Print and shaded views of the part. All mm, measured from the part's lowest x, y and z. A direction names the side the tool comes from. Round coordinates to 2 decimals unless told otherwise and drop trailing zeros. Order: outer loops, then holes, each group sorted by start corner. A loop starts at its lowest first (then second) coordinate and runs counter-clockwise, first axis right, second up. Notation, with made-up numbers: M 61.25,14 L 101.25,14 A12 cw 101.25,34 Z; hole C -38,32 d6. An arc over 180 degrees is marked long. Write each question's results on one line, items separated by ' | '. Start each with the question number.
1. Probe L1, parallel to X at y = 9.5, z = 2.5; L2, parallel to Y at x = 3.75, z = 1.25; L3, parallel to X at y = 0.2, z = 3.5 (1 decimal). List the from-to ranges inside material, lowest first. Write a range as [from, to].
2. Band-saw the part on B-B, the plane x = 5.75. List the corners of the cut face in (y, z).
3. Which spindle directions (+Z, -Z, +X, -X, +Y, -Y) get a long thin tool onto all of the face, cutting with end or side? Do the marked faces 5 and 6. Say none if no direction does.
4. Band-saw the part on D-D, the plane z = 0.5. List the corners of the cut face in (x, y).
5. Drop flat-ended pins along their axis: pin 1 Ø3.5 at (y, z) = (7, 2.5) entering from -X; pin 2 Ø3 at (x, z) = (3, 5) entering from +Y; pin 3 Ø1 at (x, y) = (6.5, 3.5) entering from +Z. Give the stop position or say it passes through.
6. Band-saw the part on C-C, the plane y = 12.25. List the corners of the cut face in (x, z).
7. Band-saw the part on A-A, the plane y = 8. List the corners of the cut face in (x, z).
8. Two-plate mould, pull along X, no slides. Class the marked faces 1, 2, 3 and 4: +X half, -X half, draft (parallel to the pull), parting line (faces both ways), or undercut.
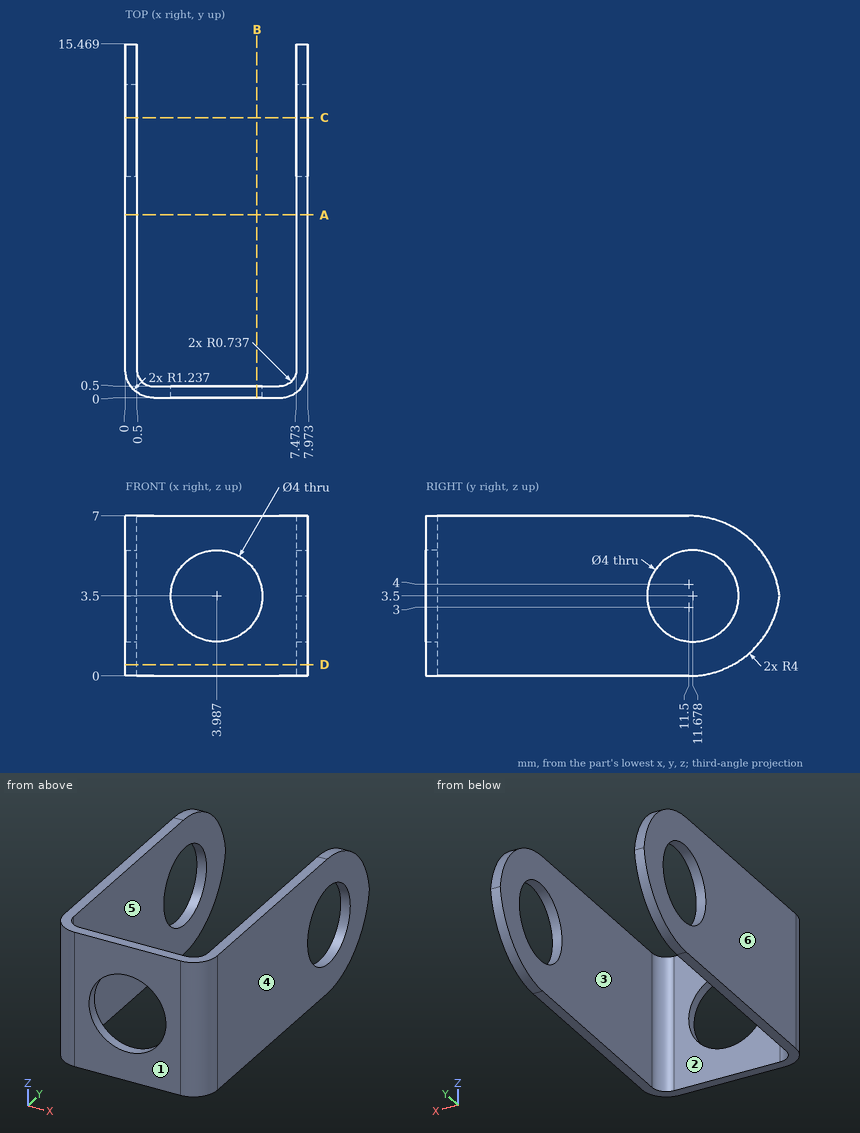
Solution:
1) L1: [0, 0.5], [7.47, 7.97] | L2: [0, 0.5] | L3: [0.6, 2], [6, 7.4]
2) outline: M 0,0 L 0.5,0 L 0.5,2.56 L 0,2.56 Z; M 0,4.44 L 0.5,4.44 L 0.5,7 L 0,7 Z
3) face 5: +Z, -Z, +Y | face 6: +Z, -Z, -X, +Y, -Y
4) outline: M 0,1.24 A1.24 ccw 1.24,0 L 6.74,0 A1.24 ccw 7.97,1.24 L 7.97,13.44 L 7.47,13.44 L 7.47,1.24 A0.74 cw 6.74,0.5 L 1.24,0.5 A0.74 cw 0.5,1.24 L 0.5,13.44 L 0,13.44 Z
5) pin 1: x = 0 | pin 2: y = 0.5 | pin 3: through
6) outline: M 0,0.07 L 0.5,0.07 L 0.5,1.58 L 0,1.58 Z; M 0,5.42 L 0.5,5.42 L 0.5,6.93 L 0,6.93 Z; M 7.47,0.07 L 7.97,0.07 L 7.97,1.58 L 7.47,1.58 Z; M 7.47,5.42 L 7.97,5.42 L 7.97,6.93 L 7.47,6.93 Z
7) outline: M 0,0 L 0.5,0 L 0.5,7 L 0,7 Z; M 7.47,0 L 7.97,0 L 7.97,7 L 7.47,7 Z
8) face 1: draft | face 2: undercut | face 3: undercut | face 4: +X half
